Autodesk Inventor part; units mm, degrees
ref_plane "YZ Plane" through (0, 0, 0) normal (1, 0, 0) x (0, 1, 0)
ref_plane "XZ Plane" through (0, 0, 0) normal (0, 1, 0) x (-1, 0, 0)
ref_plane "XY Plane" through (0, 0, 0) normal (0, 0, 1) x (1, 0, 0)
sketch "BaseI" plane through (0, 0, 0) normal (0, 0, 1) x (1, 0, 0)
  line L0 (-4.5, -10) -> (-2.65, -10)
  line L1 (5, -9.5) -> (5, 9.5)
  line L2 (4.5, 10) -> (2.65, 10)
  line L3 (-5, 9.5) -> (-5, -9.5)
  line L4 (-5, -10) -> (5, 10) construction
  line L5 (5, -10) -> (-5, 10) construction
  line L6 (3.85, 8.5) -> (2.65, 8.5)
  line L7 (-4.15, 8.2) -> (-4.15, 5.1)
  line L8 (-3.85, 4.8) -> (-2.65, 4.8)
  line L9 (4.15, 5.1) -> (4.15, 8.2)
  line L10 (4.15, 8.5) -> (-4.15, 4.8) construction
  line L11 (-4.15, 8.5) -> (4.15, 4.8) construction
  line L12 (-1.55, 3) -> (1.55, 3)
  line L13 (2.15, 3.6) -> (2.15, 4.3)
  line L14 (-2.15, 9.5) -> (-2.15, 9)
  line L15 (-2.15, 3) -> (2.15, 10) construction
  line L16 (2.15, 3) -> (-2.15, 10) construction
  line L17 (3.85, -8.5) -> (2.65, -8.5)
  line L18 (-4.15, -8.2) -> (-4.15, -5.1)
  line L19 (-3.85, -4.8) -> (-2.65, -4.8)
  line L20 (4.15, -5.1) -> (4.15, -8.2)
  line L21 (4.15, -8.5) -> (-4.15, -4.8) construction
  line L22 (-4.15, -8.5) -> (4.15, -4.8) construction
  line L23 (1.55, -3) -> (-1.55, -3)
  line L24 (-2.15, -3.6) -> (-2.15, -4.3)
  line L25 (2.15, -9.5) -> (2.15, -9)
  line L26 (2.15, -3) -> (-2.15, -10) construction
  line L27 (-2.15, -3) -> (2.15, -10) construction
  arc A0 (-4.5, 10) -> (-5, 9.5) centre (-4.5, 9.5) ccw
  arc A1 (5, 9.5) -> (4.5, 10) centre (4.5, 9.5) ccw
  arc A2 (4.5, -10) -> (5, -9.5) centre (4.5, -9.5) ccw
  arc A3 (-5, -9.5) -> (-4.5, -10) centre (-4.5, -9.5) ccw
  line L28 (-2.65, 10) -> (-4.5, 10)
  line L29 (2.65, -10) -> (4.5, -10)
  arc A4 (-3.85, 8.5) -> (-4.15, 8.2) centre (-3.85, 8.2) ccw
  arc A5 (-4.15, 5.1) -> (-3.85, 4.8) centre (-3.85, 5.1) ccw
  arc A6 (4.15, 8.2) -> (3.85, 8.5) centre (3.85, 8.2) ccw
  arc A7 (3.85, 4.8) -> (4.15, 5.1) centre (3.85, 5.1) ccw
  arc A8 (-3.85, -4.8) -> (-4.15, -5.1) centre (-3.85, -5.1) ccw
  arc A9 (-4.15, -8.2) -> (-3.85, -8.5) centre (-3.85, -8.2) ccw
  arc A10 (4.15, -5.1) -> (3.85, -4.8) centre (3.85, -5.1) ccw
  arc A11 (3.85, -8.5) -> (4.15, -8.2) centre (3.85, -8.2) ccw
  arc A12 (-2.15, 3.6) -> (-1.55, 3) centre (-1.55, 3.6) ccw
  arc A13 (1.55, 3) -> (2.15, 3.6) centre (1.55, 3.6) ccw
  arc A14 (-1.55, -3) -> (-2.15, -3.6) centre (-1.55, -3.6) ccw
  arc A15 (2.15, -3.6) -> (1.55, -3) centre (1.55, -3.6) ccw
  arc A16 (-2.15, 9.5) -> (-2.65, 10) centre (-2.65, 9.5) ccw
  arc A17 (2.65, 10) -> (2.15, 9.5) centre (2.65, 9.5) ccw
  line L30 (-2.65, 8.5) -> (-3.85, 8.5)
  line L31 (2.65, 4.8) -> (3.85, 4.8)
  line L32 (2.15, 9) -> (2.15, 9.5)
  line L33 (-2.15, 4.3) -> (-2.15, 3.6)
  line L34 (2.15, -4.3) -> (2.15, -3.6)
  line L35 (-2.15, -9) -> (-2.15, -9.5)
  line L36 (2.65, -4.8) -> (3.85, -4.8)
  line L37 (-2.65, -8.5) -> (-3.85, -8.5)
  arc A18 (-2.15, 4.3) -> (-2.65, 4.8) centre (-2.65, 4.3) ccw
  arc A19 (2.65, 4.8) -> (2.15, 4.3) centre (2.65, 4.3) ccw
  arc A20 (2.15, 9) -> (2.65, 8.5) centre (2.65, 9) ccw
  arc A21 (-2.65, 8.5) -> (-2.15, 9) centre (-2.65, 9) ccw
  arc A22 (-2.65, -4.8) -> (-2.15, -4.3) centre (-2.65, -4.3) ccw
  arc A23 (2.15, -4.3) -> (2.65, -4.8) centre (2.65, -4.3) ccw
  arc A24 (2.65, -8.5) -> (2.15, -9) centre (2.65, -9) ccw
  arc A25 (-2.15, -9) -> (-2.65, -8.5) centre (-2.65, -9) ccw
  arc A26 (-2.65, -10) -> (-2.15, -9.5) centre (-2.65, -9.5) ccw
  arc A27 (2.15, -9.5) -> (2.65, -10) centre (2.65, -9.5) ccw
  circle A28 centre (0, 0) radius 1.65
  point P0 (0, 6.65)
  point P1 (0, 6.5)
  point P2 (0, -6.65)
  point P3 (0, -6.5)
  point P4 (0, 6.5)
  point P5 (0, 10)
  point P6 (0, -6.5)
  point P7 (0, -10)
  point P8 (0, 6.65)
  point P9 (0, 10)
  point P10 (0, 6.65)
  point P11 (0, -6.65)
  point P12 (0, -10)
  point P13 (0, -6.5)
  point P14 (0, -6.65)
  point P15 (0, 6.5)
  dimension "d0" = 10
  dimension "d1" = 20
  dimension "d2" = 7
  dimension "d3" = 4.3
  dimension "d4" = 7
  dimension "d5" = 4.3
  dimension "d6" = 8.3
  dimension "d7" = 8.3
  dimension "d8" = 3.7
  dimension "d9" = 3.7
  dimension "d10" = 1.5
  dimension "d11" = 1.5
  dimension "d12" = 0.5
  dimension "d13" = 0.3
  dimension "d14" = 0.6
  dimension "d15" = 0.5
  dimension "d16" = 0.5
  dimension "d17" = 3.3
extrude "押し出し1" add sketch "BaseI" along normal blind 290
properties part number "I330" material "アルミニウム 6061"
Geometry check sheet. Reference: the model listing, model coordinates, mm. Coordinates: 2 decimals unless noted, no trailing zeros. Order: outer loops, then holes, each group sorted by start corner. A loop starts at its lowest first (then second) coordinate and runs counter-clockwise, first axis right, second up. Notation, with made-up numbers: (-26, 16) - (23, 16) arc R16 cw to (23, 20) - close; hole circle Ø10 at (-17.75, 20). An arc over 180 degrees is marked (long way). Answer in a Markdown table with one row per item. Add a question column.
1) Material ranges on line 1 along Y through (x, z) = (-2.75, 34); line 2 along Y through (x, z) = (0, 122.5); line 3 along X through (y, z) = (4.25, 74), recorded low to high. Write a range as [from, to].
2) Gauge pin test, flat end, axial feed: P1, Ø0.9, axis at x = -0.5, z = 144, coming from the -Y side. Record the tip position at first contact, or that the pin passes through.
3) Cross-section at A-A, the plane x = 0. Record the cut outline in (y, z).
Check result:
| question | item | result |
|---|---|---|
| 1 | line 1 | y = [-10, -8.5], [-4.8, 4.8], [8.5, 10] |
| 1 | line 2 | y = [-3, -1.65], [1.65, 3] |
| 1 | line 3 | x = [-5, -2.15], [2.15, 5] |
| 2 | P1 | stops at y = -3 |
| 3 | outline | (-3, 0) - (-1.65, 0) - (-1.65, 290) - (-3, 290) - close; (1.65, 0) - (3, 0) - (3, 290) - (1.65, 290) - close |
